```python
from build123d import *

# Parameters (mm, degrees)
SKETCH_R        = 3.746138
PAD_DEPTH       = 10
CHAMFER_SIZE    = 3
POCKET_DEPTH    = 1
POCKET001_DEPTH = 9.001


with BuildPart() as part:
    # Sketch → Pad (new body)
    with BuildSketch(Plane.XY):
        with BuildLine():
            ThreePointArc((-23.772092, 3.904727), (-24.696894, 0), (-23.772092, -3.904727))
            Line((-23.772092, -3.904727), (-8.931203, -37.109992))
            ThreePointArc((-8.931203, -37.109992), (0, -41.688736), (8.931203, -37.109992))
            Line((8.931203, -37.109992), (23.772092, -3.904727))
            ThreePointArc((23.772092, -3.904727), (24.696894, 0), (23.772092, 3.904727))
            Line((10.593771, 37.804188), (23.772092, 3.904727))
            ThreePointArc((10.593771, 37.804188), (0, 45.842754), (-10.593771, 37.804188))
            Line((-10.593771, 37.804188), (-23.772092, 3.904727))
        make_face()
        with Locations((0, 34.842873)):
            Circle(SKETCH_R, mode=Mode.SUBTRACT)
        with Locations((0, -30.688856)):
            Circle(SKETCH_R, mode=Mode.SUBTRACT)
    extrude(amount=PAD_DEPTH)

    # Chamfer
    chamfer_edges = [part.edges().sort_by_distance(p)[0] for p in [
        (-3.746138, 34.842873, 10),
        (-3.746138, -30.688856, 10),
    ]]
    chamfer(chamfer_edges, length=CHAMFER_SIZE)

    # Sketch001 (on Face4 of Chamfer) → Pocket (cut)
    with BuildSketch(Plane.XY.offset(10)):
        with BuildLine():
            ThreePointArc((5.49555, 17.868014), (0, 21.260344), (-5.49555, 17.868014))
            Line((-5.49555, 17.868014), (-13.141501, 2.617381))
            ThreePointArc((-13.141501, 2.617381), (-13.760876, 0), (-13.141501, -2.617381))
            Line((-13.141501, -2.617381), (-5.49555, -17.868014))
            ThreePointArc((-5.49555, -17.868014), (0, -21.260344), (5.49555, -17.868014))
            Line((5.49555, -17.868014), (13.141501, -2.617381))
            ThreePointArc((13.141501, -2.617381), (13.760876, 0), (13.141501, 2.617381))
            Line((5.49555, 17.868014), (13.141501, 2.617381))
        make_face()
    extrude(amount=-POCKET_DEPTH, mode=Mode.SUBTRACT)

    # Sketch002 (on Face23 of Pocket) → Pocket001 (cut, through all)
    with BuildSketch(Plane.XY.offset(9)):
        with BuildLine():
            ThreePointArc((-4.053463, 8.314375), (-9.249832, 0), (-4.053463, -8.314375))
            Line((-4.053463, -8.314375), (-4.053463, -13.561737))
            Line((-4.053463, -13.561737), (4.053463, -13.561737))
            Line((4.053463, -13.561737), (4.053463, -8.314375))
            ThreePointArc((4.053463, -8.314375), (9.249832, 0), (4.053463, 8.314375))
            Line((4.053463, 8.314375), (4.053463, 13.561737))
            Line((4.053463, 13.561737), (-4.053463, 13.561737))
            Line((-4.053463, 13.561737), (-4.053463, 8.314375))
        make_face()
    extrude(amount=-POCKET001_DEPTH, mode=Mode.SUBTRACT)


solid = part.part
```
For this review, take the finished solid that the model builds, in its own axes (mm). A direction names the side the tool comes from. Round coordinates to 2 decimals unless told otherwise and drop trailing zeros. Write each loop counter-clockwise with the first axis right and the second up, starting at its lowest first coordinate (ties: lowest second). Pieces come first, ordered by that corner, then holes.
1) Mouldability with a two-part tool opening along Y and no side actions: class faces 4 (the face through (9.265, 10.349, 9.507)), 5 (the face through (-0.146, -41.688, 4.93)), 6 (the face through (11, 3, 0)), 7 (the face through (-17.09, 21.09, 4.93)) as +Y half, -Y half, draft (parallel to the pull), parting line (faces both ways), or undercut.
Answer below:
face 4: undercut
face 5: -Y half
face 6: draft
face 7: +Y half
2) Take a section at C-C on z = 4.5. Give the boundary of the cut face in (x, y), then the cut area to 3 significant figures.
Answer below:
outline: (-23.77, -3.9) - (-8.93, -37.11) arc R11 ccw to (8.93, -37.11) - (23.77, -3.9) arc R8.71 ccw to (23.77, 3.9) - (10.59, 37.8) arc R11 ccw to (-10.59, 37.8) - (-23.77, 3.9) arc R8.71 ccw to start; hole (-4.05, -13.56) - (4.05, -13.56) - (4.05, -8.31) arc R9.25 ccw to (4.05, 8.31) - (4.05, 13.56) - (-4.05, 13.56) - (-4.05, 8.31) arc R9.25 ccw to (-4.05, -8.31) - close; hole circle Ø7.49 at (0, -30.69); hole circle Ø7.49 at (0, 34.84)
area: 2,380 mm2
3) Machinability: for faces 1 (the face through (-9.265, 10.349, 9.507)), 2 (the face through (-9.25, 0.14, 4.56)), 3 (the face through (-16.456, -20.275, 4.93)), which of the approach directions +Z, -Z, +X, -X, +Y, -Y give a long, thin tool a straight path to every point of the face, cutting with its end or side? Answer none if there is none.
Answer below:
face 1: +Z
face 2: +Z, -Z
face 3: +Z, -Z, -X, -Y
4) Take a section at D-D on y = 27. Give the boundary of the cut face in (x, z).
Answer below:
outline: (-14.79, 0) - (14.79, 0) - (14.79, 10) - (-14.79, 10) - close
5) Insertion check: pin 1 Ø4 at (y, z) = (-10, 5.5) entering from +X; pin 2 Ø10 at (x, y) = (9.5, -20) entering from -Z; pin 3 Ø3 at (y, z) = (28, 6) entering from -X; pin 4 Ø1.6 at (y, z) = (-10.5, 4) entering from -X. Each pin has a flat end and moves straight along its axis. Give the tip position at first contact, or say it passes through.
Answer below:
pin 1: stops at x = 21.94
pin 2: stops at z = 0
pin 3: stops at x = -14.99
pin 4: stops at x = -21.18
6) For line 1 along Y through (x, z) = (0, 4) (3 decimals); line 2 along X through (y, z) = (31.5, 1.5); line 3 along X through (y, z) = (-1, 4.75), list the stretches that pass through material, from the lowest coordinate up.
Answer below:
line 1: y = -41.689 to -34.435, -26.943 to -13.562, 13.562 to 31.097, 38.589 to 45.843
line 2: x = -13.04 to -1.69, 1.69 to 13.04
line 3: x = -24.64 to -9.2, 9.2 to 24.64
7) Take a section at A-A on x = 0. Give the boundary of the cut face in (y, z) (3 decimals), then the cut area to 3 significant figures.
Answer below:
outline: (-41.689, 0) - (-34.435, 0) - (-34.435, 7) - (-37.435, 10) - (-41.689, 10) - close; (-26.943, 0) - (-13.562, 0) - (-13.562, 9) - (-21.26, 9) - (-21.26, 10) - (-23.943, 10) - (-26.943, 7) - close; (13.562, 0) - (31.097, 0) - (31.097, 7) - (28.097, 10) - (21.26, 10) - (21.26, 9) - (13.562, 9) - close; (38.589, 0) - (45.843, 0) - (45.843, 10) - (41.589, 10) - (38.589, 7) - close
area: 421 mm2
8) Take a section at B-B on y = -9.5. Give the boundary of the cut face in (x, z).
Answer below:
outline: (-21.27, 0) - (-4.05, 0) - (-4.05, 9) - (-9.69, 9) - (-9.69, 10) - (-21.27, 10) - close; (4.05, 0) - (21.27, 0) - (21.27, 10) - (9.69, 10) - (9.69, 9) - (4.05, 9) - close
